Check sheet for the modelled part. Datum: model origin and axes. Units: mm. Face numbers are marked on the shaded views. A direction names the side the tool comes from. Round coordinates to 2 decimals unless told otherwise and drop trailing zeros. Order: outer loops, then holes, each group sorted by start corner. A loop starts at its lowest first (then second) coordinate and runs counter-clockwise, first axis right, second up. Notation, with made-up numbers: (58.5, 16) -> (98.5, 16) arc R28 ccw to (98.5, 51) -> close; hole circle Ø2 at (38.5, 22). An arc over 180 degrees is marked (long way). Answer in a Markdown table with one row per item.
Autodesk Inventor part; units mm, degrees
ref_plane "YZ Plane" through (0, 0, 0) normal (1, 0, 0) x (0, 1, 0)
ref_plane "XZ Plane" through (0, 0, 0) normal (0, 1, 0) x (-1, 0, 0)
ref_plane "XY Plane" through (0, 0, 0) normal (0, 0, 1) x (1, 0, 0)
sketch "Sketch1" plane through (0, 0, 0) normal (1, 0, 0) x (0, 1, 0)
  line L0 (-6, -12.5) -> (-6, -12.9)
  arc A0 (-6, -12.9) -> (-5.6, -13.3) centre (-5.6, -12.9) ccw
  line L1 (-5.6, -13.3) -> (-4.9, -13.3)
  arc A1 (-4.9, -13.3) -> (-4.7, -13.1) centre (-4.9, -13.1) ccw
  line L2 (-4.7, -13.1) -> (-4.7, -12.85)
  arc A2 (-4.5, -12.65) -> (-4.7, -12.85) centre (-4.5, -12.85) ccw
  line L3 (-4.5, -12.65) -> (-1.8, -12.65)
  arc A3 (-1.4, -13.05) -> (-1.8, -12.65) centre (-1.8, -13.05) ccw
  line L4 (-1.4, -13.05) -> (-1.4, -18.75)
  line L5 (-1.8, -19.15) -> (-4.5, -19.15)
  arc A4 (-1.8, -19.15) -> (-1.4, -18.75) centre (-1.8, -18.75) ccw
  arc A5 (-4.7, -18.95) -> (-4.5, -19.15) centre (-4.5, -18.95) ccw
  line L6 (-4.7, -18.95) -> (-4.7, -18.7)
  arc A6 (-4.7, -18.7) -> (-4.9, -18.5) centre (-4.9, -18.7) ccw
  line L7 (-4.9, -18.5) -> (-5.6, -18.5)
  arc A7 (-5.6, -18.5) -> (-6, -18.9) centre (-5.6, -18.9) ccw
  line L8 (-6, -18.9) -> (-6, -19.5)
  line L9 (-6.5, -6.5) -> (-6.5, -12.5)
  line L10 (-6.5, -12.5) -> (-2.5, -12.5)
  line L11 (-1.05, -19.5) -> (-6.5, -19.5)
  line L12 (-6.5, -19.5) -> (-6.5, -26)
  line L13 (-6.5, -26) -> (-1.05, -26)
  line L14 (-6, -26) -> (-6, -26.6)
  arc A8 (-6, -26.6) -> (-5.6, -27) centre (-5.6, -26.6) ccw
  line L15 (-5.6, -27) -> (-4.9, -27)
  arc A9 (-4.9, -27) -> (-4.7, -26.8) centre (-4.9, -26.8) ccw
  arc A10 (-4.5, -26.35) -> (-4.7, -26.55) centre (-4.5, -26.55) ccw
  line L16 (-4.7, -26.8) -> (-4.7, -26.55)
  line L17 (-4.5, -26.35) -> (-1.8, -26.35)
  arc A11 (-1.4, -26.75) -> (-1.8, -26.35) centre (-1.8, -26.75) ccw
  line L18 (-1.4, -26.75) -> (-1.4, -32.45)
  arc A12 (-1.8, -32.85) -> (-1.4, -32.45) centre (-1.8, -32.45) ccw
  line L19 (-1.8, -32.85) -> (-4.5, -32.85)
  arc A13 (-4.7, -32.65) -> (-4.5, -32.85) centre (-4.5, -32.65) ccw
  line L20 (-4.7, -32.65) -> (-4.7, -32.4)
  arc A14 (-4.7, -32.4) -> (-4.9, -32.2) centre (-4.9, -32.4) ccw
  line L21 (-4.9, -32.2) -> (-5.6, -32.2)
  arc A15 (-5.6, -32.2) -> (-6, -32.6) centre (-5.6, -32.6) ccw
  line L22 (-6, -32.6) -> (-6, -33)
  line L23 (-2.5, -33) -> (-6.5, -33)
  line L24 (-6.5, -33) -> (-6.5, -39)
  line L25 (32.5, 0) -> (0, 0)
  circle A16 centre (0, -6.5) radius 4.75
  circle A17 centre (32.5, -6.5) radius 4.75
  circle A18 centre (0, -39) radius 4.75
  circle A19 centre (32.5, -39) radius 4.75
  line L26 (39, -26) -> (39, -19.5)
  line L27 (39, -12.5) -> (39, -6.5)
  line L28 (39, -39) -> (39, -33)
  line L29 (26.5, -45.5) -> (32.5, -45.5)
  line L30 (0, -45.5) -> (6, -45.5)
  line L31 (13, -45.5) -> (19.5, -45.5)
  circle A20 centre (16.25, -22.75) radius 15
  circle A21 centre (16.2588, 5.0016) radius 2.5
  circle A22 centre (16.25, -50.5) radius 2.5
  circle A23 centre (16.25, -22.75) radius 5
  circle A24 centre (16.25, -22.75) radius 8.45
  line L32 (24.75, -27.6575) -> (24.75, -17.8425)
  line L33 (44, 10) -> (-11.5, 10)
  line L34 (-11.5, 10) -> (-11.5, -55.5)
  line L35 (-11.5, -55.5) -> (44, -55.5)
  line L36 (44, -55.5) -> (44, 10)
  line L37 (-11.5, 30) -> (44, 30)
  line L38 (-11.5, -75.5) -> (-11.5, 30)
  line L39 (44, 30) -> (44, -75.5)
  line L40 (44, -75.5) -> (-11.5, -75.5)
  circle A25 centre (16.25, -65.5) radius 5
  circle A26 centre (16.25, 20) radius 5
  line L41 (44, 30) -> (44, 50)
  line L42 (44, -75.5) -> (44, -95.5)
  line L43 (110, 50) -> (84, 50)
  line L44 (84, 50) -> (84, -95.5)
  line L45 (84, -95.5) -> (110, -95.5)
  line L46 (110, -95.5) -> (110, 50)
  line L47 (84, 50) -> (104, 50)
  line L48 (104, -95.5) -> (84, -95.5)
  line L49 (84, -95.5) -> (84, 50)
  line L50 (84, 50) -> (64, 50)
  line L51 (64, 50) -> (64, -95.5)
  line L52 (64, -95.5) -> (84, -95.5)
  line L53 (84, -95.5) -> (84, 50)
  line L54 (64, 50) -> (44, 50)
  line L55 (44, 50) -> (44, -95.5)
  line L56 (44, -95.5) -> (64, -95.5)
  line L57 (64, -95.5) -> (64, 50)
  line L58 (44, 30) -> (54, 30)
  line L59 (100.8097, 50) -> (100.8097, 40)
  line L60 (94, -95.5) -> (94, -85.5)
  line L61 (110, 40) -> (54, 40)
  line L62 (54, 40) -> (54, -85.5)
  line L63 (54, -85.5) -> (110, -85.5)
  line L64 (110, 50) -> (136, 50)
  line L65 (136, 50) -> (136, 40)
  line L66 (136, 40) -> (110, 40)
  line L67 (110, -85.5) -> (136, -85.5)
  line L68 (136, -85.5) -> (136, -95.5)
  line L69 (136, -95.5) -> (110, -95.5)
  dimension "d0" = 20
  dimension "d1" = 20
  dimension "d2" = 55.5
  dimension "d3" = 26
  dimension "d5" = 20
  dimension "d6" = 45.5
  dimension "d7" = 20
  dimension "d8" = 10
  dimension "d9" = 10
  dimension "d10" = 26
extrude "Extrusion1" add sketch "Sketch1" along normal blind 75.5 contours L39 L58 L62 L63 L51 L56 L42 L36 | L41 L54 L51 L61 L62 L58 | L50 L44 L61 L51 | L51 L63 L44 L52 | L43 L59 L61 L44 | L44 L63 L60 L45 | L43 L46 L61 L59 | L60 L63 L46 L45 | L64 L65 L66 L46 | L67 L68 L69 L46
sketch "Sketch2" plane through (0, 44, -95.5) normal (0, -1, 0) x (1, 0, 0)
  line L0 (15.5, 83) -> (15.5, 82.6)
  arc A0 (15.5, 82.6) -> (15.9, 82.2) centre (15.9, 82.6) ccw
  line L1 (15.9, 82.2) -> (16.6, 82.2)
  arc A1 (16.6, 82.2) -> (16.8, 82.4) centre (16.6, 82.4) ccw
  line L2 (16.8, 82.4) -> (16.8, 82.65)
  arc A2 (17, 82.85) -> (16.8, 82.65) centre (17, 82.65) ccw
  line L3 (17, 82.85) -> (19.7, 82.85)
  arc A3 (20.1, 82.45) -> (19.7, 82.85) centre (19.7, 82.45) ccw
  line L4 (20.1, 82.45) -> (20.1, 76.75)
  line L5 (19.7, 76.35) -> (17, 76.35)
  arc A4 (19.7, 76.35) -> (20.1, 76.75) centre (19.7, 76.75) ccw
  arc A5 (16.8, 76.55) -> (17, 76.35) centre (17, 76.55) ccw
  line L6 (16.8, 76.55) -> (16.8, 76.8)
  arc A6 (16.8, 76.8) -> (16.6, 77) centre (16.6, 76.8) ccw
  line L7 (16.6, 77) -> (15.9, 77)
  arc A7 (15.9, 77) -> (15.5, 76.6) centre (15.9, 76.6) ccw
  line L8 (15.5, 76.6) -> (15.5, 76)
  line L9 (15, 89) -> (15, 83)
  line L10 (15, 83) -> (19, 83)
  line L11 (20.45, 76) -> (15, 76)
  line L12 (15, 76) -> (15, 69.5)
  line L13 (15, 69.5) -> (20.45, 69.5)
  line L14 (15.5, 69.5) -> (15.5, 68.9)
  arc A8 (15.5, 68.9) -> (15.9, 68.5) centre (15.9, 68.9) ccw
  line L15 (15.9, 68.5) -> (16.6, 68.5)
  arc A9 (16.6, 68.5) -> (16.8, 68.7) centre (16.6, 68.7) ccw
  arc A10 (17, 69.15) -> (16.8, 68.95) centre (17, 68.95) ccw
  line L16 (16.8, 68.7) -> (16.8, 68.95)
  line L17 (17, 69.15) -> (19.7, 69.15)
  arc A11 (20.1, 68.75) -> (19.7, 69.15) centre (19.7, 68.75) ccw
  line L18 (20.1, 68.75) -> (20.1, 63.05)
  arc A12 (19.7, 62.65) -> (20.1, 63.05) centre (19.7, 63.05) ccw
  line L19 (19.7, 62.65) -> (17, 62.65)
  arc A13 (16.8, 62.85) -> (17, 62.65) centre (17, 62.85) ccw
  line L20 (16.8, 62.85) -> (16.8, 63.1)
  arc A14 (16.8, 63.1) -> (16.6, 63.3) centre (16.6, 63.1) ccw
  line L21 (16.6, 63.3) -> (15.9, 63.3)
  arc A15 (15.9, 63.3) -> (15.5, 62.9) centre (15.9, 62.9) ccw
  line L22 (15.5, 62.9) -> (15.5, 62.5)
  line L23 (19, 62.5) -> (15, 62.5)
  line L24 (15, 62.5) -> (15, 56.5)
  line L25 (54, 95.5) -> (21.5, 96.1203)
  circle A16 centre (21.5, 89) radius 4.75
  circle A17 centre (54, 89) radius 4.75
  circle A18 centre (21.5, 56.5) radius 4.75
  circle A19 centre (54, 56.5) radius 4.75
  line L26 (60.5, 69.5) -> (60.5, 76)
  line L27 (60.5, 83) -> (60.5, 89)
  line L28 (60.5, 56.5) -> (60.5, 62.5)
  line L29 (48, 50) -> (54, 50)
  line L30 (21.5, 50) -> (27.5, 50)
  line L31 (34.5, 50) -> (41, 50)
  circle A20 centre (37.75, 72.75) radius 15
  circle A21 centre (37.7588, 100.5016) radius 2.5
  circle A22 centre (37.75, 45) radius 2.5
  circle A23 centre (37.75, 72.75) radius 5
  circle A24 centre (37.75, 72.75) radius 8.45
  line L32 (46.25, 67.8425) -> (46.25, 77.6575)
  line L33 (65.5, 105.5) -> (10, 105.5)
  line L34 (10, 105.5) -> (10, 40)
  line L35 (10, 40) -> (65.5, 40)
  line L36 (65.5, 40) -> (65.5, 105.5)
  line L37 (10, 125.5) -> (65.5, 125.5)
  line L38 (10, 20) -> (10, 125.5)
  line L39 (65.5, 125.5) -> (65.5, 20)
  line L40 (65.5, 20) -> (10, 20)
  circle A25 centre (37.75, 30) radius 5
  circle A26 centre (37.75, 115.5) radius 5
  line L41 (0, 145.5) -> (0, 0)
  line L42 (75.5, 145.5) -> (75.5, 0)
  line L43 (0, 145.5) -> (75.5, 0)
  line L44 (75.5, 0) -> (75.5, 145.5)
  line L45 (75.5, 145.5) -> (0, 0)
  line L46 (37.75, 72.75) -> (-23.5643, 72.75)
  point P0 (0, 95.5)
extrude "Extrusion2" cut sketch "Sketch2" against normal blind 75.5 contours A25 | A26
sketch "Sketch3" plane through (0, 44, -95.5) normal (0, 0, -1) x (-1, 0, 0)
  line L0 (0, 92) -> (-75.5, 92)
  line L1 (-75.5, 92) -> (-10, 92)
  line L2 (-10, 92) -> (-10, 36.5)
  line L3 (-10, 36.5) -> (-75.5, 36.5)
  line L4 (-75.5, 36.5) -> (-75.5, 92)
  line L5 (-42.75, 36.5) -> (-42.75, 92)
  line L6 (-10, 36.5) -> (-42.75, 92)
  line L7 (-26.375, 64.25) -> (-42.75, 64.25)
  line L8 (-42.75, 36.5) -> (-75.5, 92)
  line L9 (-59.125, 64.25) -> (-42.75, 64.25)
  circle A0 centre (-26.375, 64.25) radius 5
  circle A1 centre (-59.125, 64.25) radius 5
  point P0 (0, -44)
  dimension "d21" = 65.5
  dimension "d22" = 55.5
  dimension "d23" = 10
  dimension "d24" = 10
extrude "Extrusion3" cut sketch "Sketch3" against normal through all contours A0 L6 | L6 L7 A0 | A0 L7 L6 | A1 L9 L8 | L8 A1 | A1 L8 L9
properties part number "CarroSuperior"
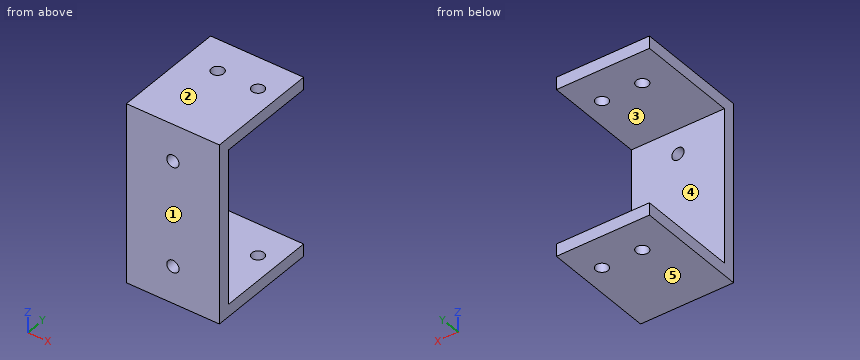
(1) Scan lines: probe 1 along Z at (x, y) = (26, 59.5); probe 2 along X at (y, z) = (50, -65); probe 3 along Y at (x, z) = (4.5, -54). Record each from-to range of solid material in increasing order. Write a range as from..to.
Solutions:
| item | result |
|---|---|
| probe 1 | -95.5..-85.5, 40..50 |
| probe 2 | 0..32.78, 42.72..75.5 |
| probe 3 | 44..54 |
(2) Depth check by flat-ended pin: pin 1 Ø4 at (x, z) = (39.5, -30.5) entering from +Y; pin 2 Ø9 at (x, z) = (37.75, -65.5) entering from -Y. Enter the tip coordinate at first touch or a pass-through.
Solutions:
| item | result |
|---|---|
| pin 1 | y = 54 |
| pin 2 | through |
(3) Section check A-A on z = -65.5. Record the boundary of the cut face in (x, y), plus the area to 3 significant figures.
Solutions:
| item | result |
|---|---|
| outline | (0, 44) -> (32.75, 44) -> (32.75, 54) -> (0, 54) -> close; (42.75, 44) -> (75.5, 44) -> (75.5, 54) -> (42.75, 54) -> close |
| area | 655 mm^2 |
(4) Tool access check on the marked faces 4 and 5. Record the directions out of +Z, -Z, +X, -X, +Y, -Y that give a thin tool (end or side, any length) a straight path to the whole face; none if there is none.
Solutions:
| item | result |
|---|---|
| face 4 | +X, -X, +Y |
| face 5 | -Z, +X, -X, +Y, -Y |
(5) Section check C-C on x = 37.75. Record the boundary of the cut face in (y, z).
Solutions:
| item | result |
|---|---|
| outline | (44, -95.5) -> (136, -95.5) -> (136, -85.5) -> (54, -85.5) -> (54, -70.5) -> (44, -70.5) -> close; (44, -60.5) -> (54, -60.5) -> (54, 15) -> (44, 15) -> close; (44, 25) -> (54, 25) -> (54, 40) -> (136, 40) -> (136, 50) -> (44, 50) -> close |
(6) Section check B-B on y = 108.25. Record the boundary of the cut face in (x, z) (3 decimals).
Solutions:
| item | result |
|---|---|
| outline | (0, -95.5) -> (21.375, -95.5) -> (21.375, -85.5) -> (0, -85.5) -> close; (0, 40) -> (21.375, 40) -> (21.375, 50) -> (0, 50) -> close; (31.375, -95.5) -> (54.125, -95.5) -> (54.125, -85.5) -> (31.375, -85.5) -> close; (31.375, 40) -> (54.125, 40) -> (54.125, 50) -> (31.375, 50) -> close; (64.125, -95.5) -> (75.5, -95.5) -> (75.5, -85.5) -> (64.125, -85.5) -> close; (64.125, 40) -> (75.5, 40) -> (75.5, 50) -> (64.125, 50) -> close |
(7) Section check D-D on y = 77. Record the boundary of the cut face in (x, z), plus the area to 3 significant figures.
Solutions:
| item | result |
|---|---|
| outline | (0, -95.5) -> (75.5, -95.5) -> (75.5, -85.5) -> (0, -85.5) -> close; (0, 40) -> (75.5, 40) -> (75.5, 50) -> (0, 50) -> close |
| area | 1,510 mm^2 |
(8) Draft check along Z on the marked faces 1, 2 and 3. Enter one of: pulls with the +Z half, pulls with the -Z half, needs draft (parallel to the pull), parting line crosses it, or undercut.
Solutions:
| item | result |
|---|---|
| face 1 | needs draft |
| face 2 | pulls with the +Z half |
| face 3 | undercut |
